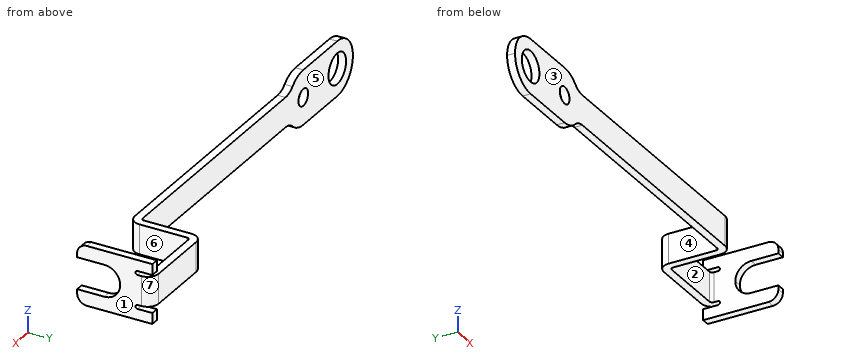
```python
from build123d import *
from build123d.topology import SkipClean

# Parameters (mm, degrees)
SKETCH_20_W                      = 0.8
SKETCH_20_H                      = 7.6
SM_BASE_FLANGE_3_DEPTH           = 3
SM_EDGE_FLANGE_4_DEPTH           = 1.9
SM_EDGE_FLANGE_4_2_DEPTH         = 1.5
SM_EDGE_FLANGE_4_3_DEPTH         = 2
SM_EDGE_FLANGE_5_STRIP_W         = 3.8
SM_EDGE_FLANGE_5_STRIP_H         = 0.8
SM_EDGE_FLANGE_5_STRIP_CUT_DEPTH = 1.5
SM_EDGE_FLANGE_5_DEPTH           = 1.5
SM_EDGE_FLANGE_6_STRIP_W         = 3.8
SM_EDGE_FLANGE_6_STRIP_H         = 0.8
SM_EDGE_FLANGE_6_STRIP_CUT_DEPTH = 1.5
SM_EDGE_FLANGE_6_DEPTH           = 1.5
SM_EDGE_FLANGE_6_PROFILE_W       = 2.75
SM_EDGE_FLANGE_6_PROFILE_H       = 37.07
SM_EDGE_FLANGE_6_FLAT_DEPTH      = 0.8
CUT_EXTRUDE_3_DEPTH              = 47.034335012
CUT_EXTRUDE_4_REACH              = 48.794
FILLET_1_R                       = 1.8
FILLET_2_R                       = 1


with BuildPart() as part:
    # 基体-法兰3: sheet metal written as solids
    # 草图20 → 基体-法兰3 (new body)
    with BuildSketch(Plane.XY):
        with Locations((0.4, 3)):
            Rectangle(SKETCH_20_W, SKETCH_20_H)
    extrude(amount=SM_BASE_FLANGE_3_DEPTH)

    # 边线-法兰4: read off the stored shape, not the designer's step
    # 边线-法兰4 outline → 边线-法兰4 (cut)
    with BuildSketch(Plane.XY):
        with BuildLine():
            Line((0, 6.8), (0, 6.758300524))
            ThreePointArc((0, 6.758300524), (0.577496438, 6.363324958), (0.8, 5.7))
            Line((0.8, 5.7), (0.8, 6.8))
            Line((0.8, 6.8), (0, 6.8))
        make_face()
    extrude(amount=SM_EDGE_FLANGE_4_DEPTH, mode=Mode.SUBTRACT)

    # Sm Edge Flange 4 2 outline → Sm Edge Flange 4 2 (add)
    with BuildSketch(Plane.XY):
        with BuildLine():
            Line((-0.3, 6.8), (-8.03, 6.8))
            Line((-8.03, 6.8), (-8.03, 6))
            Line((-8.03, 6), (-0.3, 6))
            ThreePointArc((-0.3, 6), (-0.087867966, 5.912132034), (0, 5.7))
            Line((0, 5.7), (0, 6.758300524))
            ThreePointArc((0, 6.758300524), (-0.148557894, 6.789525258), (-0.3, 6.8))
        make_face()
    extrude(amount=SM_EDGE_FLANGE_4_2_DEPTH)

    # Sm Edge Flange 4 3 outline → Sm Edge Flange 4 3 (cut)
    with BuildSketch(Plane.YZ):
        with BuildLine():
            Line((5.3, 1.5), (8, 1.5))
            Line((8, 1.5), (8, 1.9))
            Line((8, 1.9), (5.3, 1.9))
            ThreePointArc((5.3, 1.9), (5.1, 1.7), (5.3, 1.5))
        make_face()
    extrude(amount=SM_EDGE_FLANGE_4_3_DEPTH, mode=Mode.SUBTRACT)

    # 边线-法兰5: sheet metal written as solids
    # 边线-法兰5 strip (on a plane across the edge) → 边线-法兰5 strip cut (cut)
    with BuildSketch(Plane(origin=(-8.03, 6, 1.5), x_dir=(1, 0, 0), z_dir=(0, 0, -1))):
        with Locations((-0.8, -0.4)):
            Rectangle(SM_EDGE_FLANGE_5_STRIP_W, SM_EDGE_FLANGE_5_STRIP_H)
    extrude(amount=SM_EDGE_FLANGE_5_STRIP_CUT_DEPTH, mode=Mode.SUBTRACT)

    # 边线-法兰5 section (on a plane across the edge) → 边线-法兰5 (add)
    with BuildSketch(Plane(origin=(-8.03, 6, 1.5), x_dir=(1, 0, 0), z_dir=(0, 0, -1))):
        with BuildLine():
            Line((0, 0.3), (0, 6.2))
            Line((0, 6.2), (0.8, 6.2))
            Line((0.8, 6.2), (0.8, 0.3))
            ThreePointArc((0.8, 0.3), (0.887867966, 0.087867966), (1.1, 0))
            Line((1.1, 0), (1.1, -0.8))
            ThreePointArc((1.1, -0.8), (0.322182541, -0.477817459), (0, 0.3))
        make_face()
    extrude(amount=SM_EDGE_FLANGE_5_DEPTH)

    # 边线-法兰6: sheet metal written as solids
    # 边线-法兰6 strip (on a plane across the edge) → 边线-法兰6 strip cut (cut)
    with BuildSketch(Plane(origin=(-8.03, -0.2, 0), x_dir=(0, 1, 0), z_dir=(0, 0, 1))):
        with Locations((-0.8, -0.4)):
            Rectangle(SM_EDGE_FLANGE_6_STRIP_W, SM_EDGE_FLANGE_6_STRIP_H)
    extrude(amount=SM_EDGE_FLANGE_6_STRIP_CUT_DEPTH, mode=Mode.SUBTRACT)

    # 边线-法兰6 bend section (on a plane across the edge) → 边线-法兰6 (add)
    with BuildSketch(Plane(origin=(-8.03, -0.2, 0), x_dir=(0, 1, 0), z_dir=(0, 0, 1))):
        with BuildLine():
            Line((0, 0.3), (0.8, 0.3))
            ThreePointArc((0.8, 0.3), (0.887867966, 0.087867966), (1.1, 0))
            Line((1.1, 0), (1.1, -0.8))
            ThreePointArc((1.1, -0.8), (0.322182541, -0.477817459), (0, 0.3))
        make_face()
    extrude(amount=SM_EDGE_FLANGE_6_DEPTH)

    # 边线-法兰6 profile (on flange) → 边线-法兰6 flat (add)
    with BuildSketch(Plane(origin=(-8.03, -0.2, 0), x_dir=(0, 0, 1), z_dir=(0, -1, 0))):
        with Locations((1.375, 18.835)):
            Rectangle(SM_EDGE_FLANGE_6_PROFILE_W, SM_EDGE_FLANGE_6_PROFILE_H)
    extrude(amount=-SM_EDGE_FLANGE_6_FLAT_DEPTH)

    # 草图37 → 切除-拉伸3 (cut, through all)
    with BuildSketch(Plane.XZ.offset(0.2)):
        with BuildLine():
            Line((-34.345113886, 1.5), (-8.33, 1.5))
            Line((-8.33, 1.5), (-8.33, 2.75))
            Line((-8.33, 2.75), (-36.65, 2.75))
            ThreePointArc((-36.65, 2.75), (-35.33898894, 2.417384951), (-34.345113886, 1.5))
        make_face()
        with BuildLine():
            Line((-37.5, 0), (-35.8, 0))
            ThreePointArc((-35.8, 0), (-36.65, 0.85), (-37.5, 0))
        make_face()
        with BuildLine():
            ThreePointArc((-45.4, 0), (-44.594543648, 1.944543648), (-42.65, 2.75))
            Line((-42.65, 2.75), (-45.4, 2.75))
            Line((-45.4, 2.75), (-45.4, 0))
        make_face()
        with BuildLine():
            Line((-44.2, 0), (-41.1, 0))
            ThreePointArc((-41.1, 0), (-42.65, 1.55), (-44.2, 0))
        make_face()
    extrude(amount=-CUT_EXTRUDE_3_DEPTH, mode=Mode.SUBTRACT)

    # 草图38 → 切除-拉伸4 (cut, up to next)
    with BuildSketch(Plane(origin=(0.8, 0, 0), x_dir=(0, 0, -1), z_dir=(1, 0, 0)), mode=Mode.PRIVATE) as cut_extrude_4_sk1:
        with BuildLine():
            Line((-1.6, 1.95), (-1.6, -0.8))
            Line((-1.6, -0.8), (0, -0.8))
            Line((0, -0.8), (0, 3.55))
            ThreePointArc((0, 3.55), (-1.13137085, 3.08137085), (-1.6, 1.95))
        make_face()
    cut_extrude_4_tool1 = extrude(cut_extrude_4_sk1.sketch, amount=-CUT_EXTRUDE_4_REACH, mode=Mode.PRIVATE) & part.part
    add(cut_extrude_4_tool1.solids().sort_by_distance((0.8, 1.219233, 0.762069))[0], mode=Mode.SUBTRACT)

    # 圆角1
    fillet_1_edges = [part.edges().sort_by_distance(p)[0] for p in [
        (-34.345113886, 0.2, 1.5),
    ]]
    fillet(fillet_1_edges, radius=FILLET_1_R)

    # 圆角2
    fillet_2_edges = [part.edges().sort_by_distance(p)[0] for p in [
        (0.4, -0.8, 3),
    ]]
    fillet(fillet_2_edges, radius=FILLET_2_R)

    # 镜向1: part across plane


with BuildPart() as part_1:
    with SkipClean():  # the faces are left unmerged after this step: merging them gives an invalid solid
        add(part.part)
        add(part.part.mirror(Plane(origin=(-8.03, -0.2, 0), x_dir=(1, 0, 0), z_dir=(0, 0, 1))))


solid = part_1.part
```
Model file for the job. Use its own axes, mm. Face numbers are marked on the shaded views. A direction names the side the tool comes from. Coordinates: 2 decimals unless noted, no trailing zeros. Loops run counter-clockwise (first coordinate to the right, second up) from the corner with the lowest first, then second, coordinate; pieces in that order, holes last. Notation, with made-up numbers: (-24, 78.5) -> (-5, 78.5) arc R22 cw to (-5, 110.5) -> close; hole circle Ø11 at (28.25, 19.5). An arc over 180 degrees is marked (long way). Answer as a JSON object with one key per item and string values.
Q1. Flat gauge pins, fed straight in: P1, Ø3, axis at y = 2, z = -1, coming from the -X side; P2, Ø2, axis at x = -8.5, y = 2, coming from the -Z side; P3, Ø3.5, axis at y = 4, z = 0.5, coming from the -X side. Where does each tip first touch, or does it go through?
Report:
{"P1": "stops at x = -45.36", "P2": "stops at z = -1.5", "P3": "stops at x = -8.03"}
Q2. 3-axis set-ups, long thin cutter, end or side, ignore diameter. For the marked faces 1, 2, 3 and 4: which of +Z, -Z, +X, -X, +Y, -Y reach the whole face in a straight line?
Report:
{"face 1": "+Z, -Z, +X, +Y, -Y", "face 2": "+Z, -Z, -Y", "face 3": "+Z, -Z, -X, -Y", "face 4": "+Z, -Z, -X, +Y"}
Q3. Pull direction X, two halves, no side cores. Call the marked faces 5, 6 and 7: released by +X, released by -X, zero draft, split by the parting line, or undercut.
Report:
{"face 5": "zero draft", "face 6": "undercut", "face 7": "released by +X"}
Q4. Cut at A-A (y = 4.5). List the corners of the cut face in (x, z), and give its area (3 significant figures).
Report:
{"outline": "(-8.03, -1.5) -> (-7.23, -1.5) -> (-7.23, 1.5) -> (-8.03, 1.5) -> close; (0, -3) -> (0.8, -3) -> (0.8, 3) -> (0, 3) -> close", "area": "7.20 mm2"}
Q5. Cut at B-B (x = -18). List the corners of the cut face in (y, z), and give its area (3 significant figures).
Report:
{"outline": "(-0.2, -1.5) -> (0.6, -1.5) -> (0.6, 1.5) -> (-0.2, 1.5) -> close", "area": "2.40 mm2"}
Q6. Probe probe 1 along Z at (x, y) = (-36.65, 0.1); probe 2 along X at (y, z) = (0.4, 0); probe 3 along Z at (x, y) = (-42.65, 0). List the from-to ranges inside material, lowest first.
Report:
{"probe 1": "z = -2.75 to -0.85, 0.85 to 2.75", "probe 2": "x = -45.4 to -44.2, -41.1 to -37.5, -35.8 to -7.35", "probe 3": "z = -2.75 to -1.55, 1.55 to 2.75"}
